```python
from build123d import *

# Parameters (mm, degrees)
F0_R     = 12.5
F0_R_2   = 6
F1_DEPTH = 25
F2_R     = 9.5
F3_DEPTH = 10
F4_W     = 32.378687
F4_H     = 14.496426
F5_DEPTH = 10


with BuildPart() as f1:
    # F0 (on Front) → F1 (new body)
    with BuildSketch(Plane.XZ):
        Circle(F0_R)
        Circle(F0_R_2, mode=Mode.SUBTRACT)
    extrude(amount=F1_DEPTH)

    # F2 (on Front) → F3 (cut)
    with BuildSketch(Plane.XZ):
        Circle(F2_R)
    extrude(amount=F3_DEPTH, mode=Mode.SUBTRACT)

    # F4 (on face) → F5 (cut)
    with BuildSketch(Plane(origin=(0, 0, 0), x_dir=(-1, 0, 0), z_dir=(0, 1, 0))):
        with Locations((-0.849587, -7.248213)):
            Rectangle(F4_W, F4_H)
    extrude(amount=-F5_DEPTH, mode=Mode.SUBTRACT)


solid = f1.part
```
Geometry check sheet. Reference: the model listing, model coordinates, mm. A direction names the side the tool comes from. Give positions to 0.01 mm unless a question says otherwise; leave off trailing zeros. Order: outer loops, then holes, each group sorted by start corner. A loop starts at its lowest first (then second) coordinate and runs counter-clockwise, first axis right, second up.
1. Section check B-B, the plane z = -5. Enter the section's corners in (x, y).
2. Section check D-D, the plane x = 5.5. Enter the section's corners in (y, z).
3. Section check C-C, the plane y = -16.5. Enter the section's corners in (x, z), and give its area (3 significant figures).
4. Thickness scan on L1, parallel to Z at x = 0, y = -15; L2, parallel to Y at x = 8.75, z = 2; L3, parallel to X at y = -16, z = -4.25. Record the ranges inside material, lowest first.
5. Release check for a two-part mould opening along Z. For faces 1 (the face through (-6, -17, 0)), 2 (the face through (0.2, -10, -6.2)), 3 (the face through (-11, -5, 0)), 4 (the face through (-1.627, -15.103, 12.394)) record: pulls with the +Z half, pulls with the -Z half, needs draft (parallel to the pull), parting line crosses it, or undercut.
6. Gauge pin test, flat ends, axial feed: pin 1 Ø5 at (y, z) = (-11, 9) entering from -X; pin 2 Ø0.9 at (x, y) = (-10.5, -2.5) entering from -Z; pin 3 Ø5 at (x, y) = (4.5, -19.5) entering from +Z; pin 4 Ø9.5 at (x, z) = (0, 0) entering from -Y. Record the tip position at first contact, or that the pin passes through.
7. Access from +Z, -Z, +X, -X, +Y, -Y to the whole of each face (thin tool, end or side, straight path). Record for faces 5 (the face through (0.209, -4.93, 9.498)), 6 (the face through (11, -5, 0)), 7 (the face through (-3, -25, -5.4)).
8. Section check A-A, the plane x = 0. Enter the section's corners in (y, z), and give its area (3 significant figures).
Values follow:
1. outline: (-11.46, -25) - (-3.32, -25) - (-3.32, -10) - (-11.46, -10) - close; (3.32, -25) - (11.46, -25) - (11.46, -10) - (3.32, -10) - close
2. outline: (-25, -11.22) - (-10, -11.22) - (-10, -2.4) - (-25, -2.4) - close; (-25, 2.4) - (-10, 2.4) - (-10, 7.75) - (0, 7.75) - (0, 11.22) - (-25, 11.22) - close
3. outline: circle Ø25 at (0, 0); hole circle Ø12 at (0, 0)
3. area: 378 mm2
4. L1: z = -12.5 to -6, 6 to 12.5
4. L2: y = -25 to -10
4. L3: x = -11.76 to -4.24, 4.24 to 11.76
5. face 1: undercut
5. face 2: needs draft
5. face 3: pulls with the -Z half
5. face 4: parting line crosses it
6. pin 1: stops at x = -10.68
6. pin 2: stops at z = 0
6. pin 3: stops at z = 12.34
6. pin 4: passes through
7. face 5: -Z, +Y
7. face 6: -Z, +X, -X, +Y
7. face 7: +Z, -Z, +X, -X, -Y
8. outline: (-25, -12.5) - (-10, -12.5) - (-10, -6) - (-25, -6) - close; (-25, 6) - (-10, 6) - (-10, 9.5) - (0, 9.5) - (0, 12.5) - (-25, 12.5) - close
8. area: 225 mm2
